CAD build for the part. Positions are in the model's coordinates, mm. A direction names the side the tool comes from. Give positions to 0.01 mm unless a question says otherwise; leave off trailing zeros. Write each loop counter-clockwise with the first axis right and the second up, starting at its lowest first coordinate (ties: lowest second). Pieces come first, ordered by that corner, then holes. Notation, with made-up numbers: (73.5, 9.5) -> (113.5, 9.5) arc R21 cw to (113.5, 18.5) -> close; hole circle Ø8 at (-22.75, 62). An arc over 180 degrees is marked (long way). Answer as a JSON object with one key per item and string values.
```python
from build123d import *

# Parameters (mm, degrees)
F0_R     = 12.87
F1_DEPTH = 40
F3_DEPTH = 15
F4_R     = 2
F5_DEPTH = 6


with BuildPart() as f1:
    # F0 (on Right) → F1 (new body)
    with BuildSketch(Plane.YZ):
        Circle(F0_R)
    extrude(amount=-F1_DEPTH)

    # F2 (on Front) → F3 (cut, symmetric)
    with BuildSketch(Plane.XZ):
        Polygon((-14.022035, -13.172213), (-40.083185, 12.888939), (-40.083185, -13.172213), align=None)
    extrude(amount=F3_DEPTH, both=True, mode=Mode.SUBTRACT)

    # F4 (on face) → F5 (join)
    with BuildSketch(Plane.YZ):
        Circle(F4_R)
    extrude(amount=F5_DEPTH)


solid = f1.part
```
1) Slice it at D-D (z = 3.75). List the corners of the cut face in (x, y), then the cut area to 3 significant figures.
Model answer:
{"outline": "(-30.94, -12.31) -> (0, -12.31) -> (0, 12.31) -> (-30.94, 12.31) -> close", "area": "762 mm2"}
2) Pin check, flat tips, straight feed: pin 1 (2 mm diameter, centred on x = -28, y = -7, fed in from +Z); pin 2 (5 mm diameter, centred on x = -7.5, z = 7.5, fed in from -Y); pin 3 (1.5 mm diameter, centred on y = 8, z = -4.5, fed in from +X). Stop position of each tip, or through.
Model answer:
{"pin 1": "stops at z = 11.39", "pin 2": "stops at y = -11.86", "pin 3": "stops at x = 0"}
3) Slice it at A-A (y = 0). List the corners of the cut face in (x, z).
Model answer:
{"outline": "(-40, 12.81) -> (-14.32, -12.87) -> (0, -12.87) -> (0, -2) -> (6, -2) -> (6, 2) -> (0, 2) -> (0, 12.87) -> (-40, 12.87) -> close"}
4) 3-axis set-ups, long thin cutter, end or side, ignore diameter. For faces 1 (the cylindrical face through (3, 0, -2)), 2 (the cylindrical face through (-15.28, -1.68, 12.76)): which of +Z, -Z, +X, -X, +Y, -Y reach the whole face in a straight line?
Model answer:
{"face 1": "+X", "face 2": "+X, -X"}
5) Slice it at C-C (x = -15.5). List the corners of the cut face in (y, z).
Model answer:
{"outline": "(-5.37, -11.69) -> (5.37, -11.69) arc R12.87 ccw (long way) to start"}
6) Wall check: probe 1 along X at (y, z) = (10, -0.25); probe 2 along Y at (x, z) = (-28.5, 7); probe 3 along Z at (x, y) = (-36, 2). Give the ranges that are in metal, low to high.
Model answer:
{"probe 1": "x = -26.94 to 0", "probe 2": "y = -10.8 to 10.8", "probe 3": "z = 8.81 to 12.71"}
7) Slice it at B-B (z = 0). List the corners of the cut face in (x, y), then the cut area to 3 significant figures.
Model answer:
{"outline": "(-27.19, -12.87) -> (0, -12.87) -> (0, -2) -> (6, -2) -> (6, 2) -> (0, 2) -> (0, 12.87) -> (-27.19, 12.87) -> close", "area": "724 mm2"}
